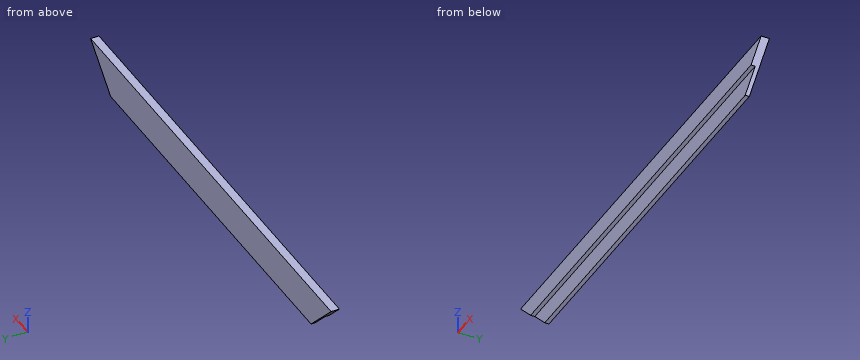
from build123d import *

# Parameters (mm, degrees)
F0_W     = 1066.8
F0_H     = 88.9
F1_DEPTH = 19.05
F2_W     = 9.525
F2_H     = 44.45
F3_DEPTH = 1066.801
F5_DEPTH = 19.051


with BuildPart() as f1:
    # F0 (on Front) → F1 (new body)
    with BuildSketch(Plane.XZ):
        with Locations((0, 44.45)):
            Rectangle(F0_W, F0_H)
    extrude(amount=F1_DEPTH)

    # F2 (on face) → F3 (cut, through all)
    with BuildSketch(Plane.YZ.offset(533.4)):
        with Locations((-14.2875, 22.225)):
            Rectangle(F2_W, F2_H)
    extrude(amount=-F3_DEPTH, mode=Mode.SUBTRACT)

    # F4 (on face) → F5 (cut, through all)
    with BuildSketch(Plane(origin=(0, 0, 0), x_dir=(-1, 0, 0), z_dir=(0, 1, 0))):
        Polygon((-444.5, 0), (-533.4, 88.9), (-533.4, 0), align=None)
        Polygon((444.5, 0), (533.4, 0), (533.4, 88.9), align=None)
    extrude(amount=-F5_DEPTH, mode=Mode.SUBTRACT)


solid = f1.part
Design review of the part built by this model. Coordinates are the model's own, in mm. Give positions to 0.01 mm unless a question says otherwise; leave off trailing zeros. Order: outer loops, then holes, each group sorted by start corner. A loop starts at its lowest first (then second) coordinate and runs counter-clockwise, first axis right, second up. Notation, with made-up numbers: (-32.75, -31.75) - (-7.75, -31.75) arc R15 cw to (-7.75, -22.75) - close; hole circle Ø6 at (-28.75, 67.25). An arc over 180 degrees is marked (long way). Use CSV: the item, a comma, the result in double quotes. Start each with the question number.
Q1. For line 1 (Z direction, x = -410.5, y = -14); line 2 (Y direction, x = -226, z = 20.5) (3 decimals); line 3 (X direction, y = -12, z = 69.5), list the stretches that pass through material, from the lowest coordinate up.
Q2. Take a section at A-A (x = 363). State the section outline as (y, z) points (3 decimals), and give its area (3 significant figures).
Q3. For P1, Ø1, axis at y = -5, z = 61, coming from the -X side; P2, Ø8, axis at y = -14.5, z = 49.5, coming from the +X side; P3, Ø2, axis at y = -11.5, z = 48, coming from the -X side, all flat-tipped, find the tip position at first contact; note any pin that passes through.
Q4. Take a section at C-C (y = -16). State the section outline as (x, z) points.
Q5. Take a section at B-B (z = 79.5). State the section outline as (x, y) points.
Calculated:
1,line 1,"z = 44.45 to 88.9"
1,line 2,"y = -9.525 to 0"
1,line 3,"x = -514 to 514"
2,outline,"(-19.05, 44.45) - (-9.525, 44.45) - (-9.525, 0) - (0, 0) - (0, 88.9) - (-19.05, 88.9) - close"
2,area,"1,270 mm²"
3,P1,"stops at x = -506"
3,P2,"stops at x = 498"
3,P3,"stops at x = -493.5"
4,outline,"(-533.4, 88.9) - (-488.95, 44.45) - (488.95, 44.45) - (533.4, 88.9) - close"
5,outline,"(-524, -19.05) - (524, -19.05) - (524, 0) - (-524, 0) - close"
